```python
from build123d import *

# Parameters (mm, degrees)
F1_DEPTH = 2.5
F3_DEPTH = 2.501


with BuildPart() as f1:
    # F0 (on Top) → F1 (new body)
    with BuildSketch(Plane.XY):
        with BuildLine():
            ThreePointArc((-11.3773406915, 13.5589866432), (-12.4804717144, 13.1173744075), (-13.5764501988, 13.5764501988))
            ThreePointArc((-13.5764501988, 13.5764501988), (-17.7384870242, 7.3475219014), (-19.2, 0))
            ThreePointArc((-19.2, 0), (-18.1004105765, -0.4503582132), (-17.6326461562, -1.5426566466))
            ThreePointArc((-17.6326461562, -1.5426566466), (-16.3526677254, -6.7734967529), (-13.5589866432, -11.3773406915))
            ThreePointArc((-13.5589866432, -11.3773406915), (-13.1173744075, -12.4804717144), (-13.5764501988, -13.5764501988))
            ThreePointArc((-13.5764501988, -13.5764501988), (-7.3475219014, -17.7384870242), (0, -19.2))
            ThreePointArc((0, -19.2), (0.4503582132, -18.1004105765), (1.5426566466, -17.6326461562))
            ThreePointArc((1.5426566466, -17.6326461562), (6.7734967529, -16.3526677254), (11.3773406915, -13.5589866432))
            ThreePointArc((11.3773406915, -13.5589866432), (12.4804717144, -13.1173744075), (13.5764501988, -13.5764501988))
            ThreePointArc((13.5764501988, -13.5764501988), (17.7384870242, -7.3475219014), (19.2, 0))
            ThreePointArc((19.2, 0), (18.1005373282, 0.4504869942), (17.6326461562, 1.5426566466))
            ThreePointArc((17.6326461562, 1.5426566466), (16.3526677254, 6.7734967529), (13.5589866432, 11.3773406915))
            ThreePointArc((13.5589866432, 11.3773406915), (13.1173744075, 12.4804717144), (13.5764501988, 13.5764501988))
            ThreePointArc((13.5764501988, 13.5764501988), (7.3475219014, 17.7384870242), (0, 19.2))
            ThreePointArc((0, 19.2), (-0.4504869942, 18.1005373282), (-1.5426566466, 17.6326461562))
            ThreePointArc((-1.5426566466, 17.6326461562), (-6.7734967529, 16.3526677254), (-11.3773406915, 13.5589866432))
        make_face()
        with BuildLine():
            ThreePointArc((15.6900664949, -1.3727029483), (14.5511026371, -6.0272640598), (12.0651999791, -10.1239048526))
            ThreePointArc((12.0651999791, -10.1239048526), (11.0599850614, -10.5489862891), (10.0762716319, -10.0762716319))
            ThreePointArc((10.0762716319, -10.0762716319), (5.4532389112, -13.1652833383), (0, -14.25))
            ThreePointArc((0, -14.25), (-0.3613316509, -15.2798492672), (-1.3727029483, -15.6900664949))
            ThreePointArc((-1.3727029483, -15.6900664949), (-6.0272640598, -14.5511026371), (-10.1239048526, -12.0651999791))
            ThreePointArc((-10.1239048526, -12.0651999791), (-10.5489862891, -11.0599850614), (-10.0762716319, -10.0762716319))
            ThreePointArc((-10.0762716319, -10.0762716319), (-13.1652833383, -5.4532389112), (-14.25, 0))
            ThreePointArc((-14.25, 0), (-15.2798501764, 0.3613306971), (-15.6900664949, 1.3727029483))
            ThreePointArc((-15.6900664949, 1.3727029483), (-14.5511026371, 6.0272640598), (-12.0651999791, 10.1239048526))
            ThreePointArc((-12.0651999791, 10.1239048526), (-11.0599850614, 10.5489862891), (-10.0762716319, 10.0762716319))
            ThreePointArc((-10.0762716319, 10.0762716319), (-5.4532389112, 13.1652833383), (0, 14.25))
            ThreePointArc((0, 14.25), (0.3613306971, 15.2798501764), (1.3727029483, 15.6900664949))
            ThreePointArc((1.3727029483, 15.6900664949), (6.0272640598, 14.5511026371), (10.1239048526, 12.0651999791))
            ThreePointArc((10.1239048526, 12.0651999791), (10.5489862891, 11.0599850614), (10.0762716319, 10.0762716319))
            ThreePointArc((10.0762716319, 10.0762716319), (13.1652833383, 5.4532389112), (14.25, 0))
            ThreePointArc((14.25, 0), (15.2798501764, -0.3613306971), (15.6900664949, -1.3727029483))
        make_face(mode=Mode.SUBTRACT)
    extrude(amount=F1_DEPTH)

    # F2 (on Top) → F3 (cut, through all)
    with BuildSketch(Plane.XY):
        with BuildLine():
            Line((-18.5884346953, 4.8072960778), (-15.248325336, 3.9434850639))
            ThreePointArc((-15.248325336, 3.9434850639), (-14.5511026371, 6.0272640598), (-13.570659277, 7.9937292166))
            Line((-13.570659277, 7.9937292166), (-16.5432798805, 9.7447365688))
            ThreePointArc((-16.5432798805, 9.7447365688), (-17.7384870242, 7.3475219014), (-18.5884346953, 4.8072960778))
        make_face()
    extrude(amount=F3_DEPTH, mode=Mode.SUBTRACT)


solid = f1.part
```
Here's how the part is built. I have some questions about the finished solid (model axes, mm). A direction names the side the tool comes from. Coordinates: 2 decimals unless noted, no trailing zeros. Order: outer loops, then holes, each group sorted by start corner. A loop starts at its lowest first (then second) coordinate and runs counter-clockwise, first axis right, second up. Notation, with made-up numbers: M -27.75,-22 L 16.25,-22 A29 ccw 16.25,14 Z; hole C -35.5,83.5 d1. An arc over 180 degrees is marked long. Answer as a JSON object with one key per item and string values. Group by question number.
(1) Suppose I cut it at A-A, the plane x = -2. Please give me the cut outline in (y, z).
(2) If we mould it in two halves opening along X, with no side actions, what happens to faces 3 (the face through (-0.35, -15.27, 1.23)), 4 (the face through (-13.117, -12.463, 1.232)), 5 (the face through (0.44, -18.11, 1.23))? For each: released by +X, released by -X, zero draft, split by the parting line, or undercut.
(3) I need wall thicknesses on probe 1 along Y at (x, z) = (-13, 0.45); probe 2 along Y at (x, z) = (-3.5, 1.25); probe 3 along X at (y, z) = (-8, 0.6). Which ranges of each line are inside material? Lowest first, please.
(4) Suppose I cut it at D-D, the plane y = 6. Please give me the cut outline in (x, z), then the cut area to 3 significant figures.
(5) Suppose I cut it at C-C, the plane x = -17. Please give me the cut outline in (y, z).
(6) Suppose I cut it at B-B, the plane y = -9. Please give me the cut outline in (x, z), then the cut area to 3 significant figures.
(7) Which directions (+Z, -Z, +X, -X, +Y, -Y) give clear straight access to the entire face, cutting with the end or side of a thin tool? Please do faces 1 (the face through (-16.94, 4.38, 1.23)), 2 (the face through (6.704, -16.381, 1.232)).
Values found:
{
 "1": {"outline": "M -19.1,0 L -15.62,0 L -15.62,2.5 L -19.1,2.5 Z; M 14.11,0 L 17.59,0 L 17.59,2.5 L 14.11,2.5 Z"},
 "2": {"face 3": "undercut", "face 4": "released by -X", "face 5": "released by +X"},
 "3": {"probe 1": "y = -14.13 to -5.84, 8.89 to 13.21", "probe 2": "y = -18.88 to -15.36, 13.81 to 17.35", "probe 3": "x = -15.79 to -11.79, 13.57 to 17.45"},
 "4": {"outline": "M 12.93,0 L 16.65,0 L 16.65,2.5 L 12.93,2.5 Z", "area": "9.32 mm^2"},
 "5": {"outline": "M -4.93,0 L 4.4,0 L 4.4,2.5 L -4.93,2.5 Z"},
 "6": {"outline": "M -15.24,0 L -11.05,0 L -11.05,2.5 L -15.24,2.5 Z; M 12.93,0 L 16.96,0 L 16.96,2.5 L 12.93,2.5 Z", "area": "20.6 mm^2"},
 "7": {"face 1": "+Z, -Z", "face 2": "+Z, -Z, +X, -Y"}
}
